Could you check a few things on this model? Use its own coordinates, in mm. A direction names the side the tool comes from. Round coordinates to 2 decimals unless told otherwise and drop trailing zeros. Write each loop counter-clockwise with the first axis right and the second up, starting at its lowest first coordinate (ties: lowest second). Pieces come first, ordered by that corner, then holes.
Autodesk Fusion 360 part; units mm, degrees
sketch "Sketch1" plane through (0, 0, 0) normal (0, 0, 1) x (1, 0, 0)
  circle A0 centre (0, 0) radius 10
  line L0 (-12.5, 12.5) -> (12.5, 12.5)
  line L1 (12.5, 12.5) -> (12.5, -12.5)
  line L2 (12.5, -12.5) -> (-12.5, -12.5)
  line L3 (-12.5, -12.5) -> (-12.5, 12.5)
  line L4 (-12.5, 6.25) -> (12.5, 6.25)
  line L5 (12.5, 6.25) -> (12.5, -6.25)
  line L6 (12.5, -6.25) -> (-12.5, -6.25)
  line L7 (-12.5, -6.25) -> (-12.5, 6.25)
  circle A1 centre (0, 0) radius 5
  dimension "d1" = 20
  dimension "d2" = 25
  dimension "d3" = 25
  dimension "d4" = 12.5
  dimension "d5" = 12.5
  dimension "d6" = 25
  dimension "d7" = 12.5
  dimension "d8" = 6.25
  dimension "d9" = 10
extrude "Extrude1" add sketch "Sketch1" along normal blind 40 contours A0 L4 | A0 L0 L1 L3 L4 | A0 L1 L2 L3 L6 | A0 L6 makes body 1 at (-4.1667, 6.25, 13.3333) makes body 2 at (4.1667, -6.25, 13.3333)
extrude "Extrude2" add sketch "Sketch1" against normal blind 20 contours A0 L4 L6 | A0 L4 | A0 L6 bodies 1 2
extrude "Extrude3" add sketch "Sketch1" along normal blind 10 contours A0 L4 L6 | A0 L1 L4 L5 L6 | A0 L3 L4 L6 L7 bodies 1
sketch "Sketch2" plane through (0, 12.5, 0) normal (0, 1, 0) x (-1, 0, 0)
  line L0 (-12.5, 0) -> (12.5, 0)
  line L1 (12.5, 0) -> (12.5, 40)
  line L2 (12.5, 40) -> (-12.5, 40)
  line L3 (-12.5, 40) -> (-12.5, 0)
  circle A0 centre (0, 27.5) radius 5
  line L4 (12.5, 0) -> (-12.5, 0)
  dimension "d16" = 10
  dimension "d17" = 27.5
extrude "Extrude4" cut sketch "Sketch2" against normal up to surface (25 mm away) contours A0 bodies 1
fillet "Fillet1" radius 12.5 4 edges at (12.5, 9.375, 40) (-12.5, 9.375, 40) (-12.5, -9.375, 40) (12.5, -9.375, 40) on bodies 1
equation "d4 = ( 25 / 2 ) * 1 mm"
equation "d5 = ( 25 / 2 ) * 1 mm"
equation "d8 = ( 12.5 / 2 ) * 1 mm"
Q1. On a 3-axis mill with a long thin cutter (end or side, diameter ignored), from which of +Z, -Z, +X, -X, +Y, -Y can I reach the whole of each face in a straight line? I mean faces 4 (the cylindrical face through (-2.17, -9.76, -9.86)), 5 (the flat face through (0, 6.25, 21)), 6 (the cylindrical face through (-8.94, -9.33, 36.24)). Say none if no direction works.
Q2. Imagine slicing it at D-D, the plane x = -7.5. Write out the boundary of the cut face in (y, z).
Q3. Imagine slicing it at B-B, the plane z = 11.5. Write out the boundary of the cut face in (x, y), then the cut area to 4 significant figures.
Q4. We'd pull the mould along Y, two halves only. Please class faces 1 (the cylindrical face through (8.94, 9.33, 36.24)), 2 (the flat face through (0, -12.5, 20)), 3 (the cylindrical face through (-1.08, 4.88, -5.21)): pulls with the +Y half, pulls with the -Y half, needs draft (parallel to the pull), parting line crosses it, or undercut.
Q5. I'm going to push flat-ended pins straight in: pin 1 Ø12 at (x, z) = (3.5, -4.5) entering from +Y; pin 2 Ø3 at (x, y) = (-3, 2) entering from +Z. Where does each tip first touch, or does it pass through?
Q6. Imagine slicing it at C-C, the plane z = 29. Write out the boundary of the cut face in (x, y).
Q7. If I drill on L1, parallel to Y at x = 2.5, z = 10.5; L2, parallel to Z at x = 0, y = -7.75; L3, parallel to Z at x = 11.5, y = 0.5, over which ranges is the centre line in solid material (lowest first)?
Q8. Imagine slicing it at A-A, the plane y = 0. Write out the boundary of the cut face in (x, z), then the cut area to 3 significant figures.
Results found:
1. face 4: -Z
1. face 5: +Z, +X, -X
1. face 6: +Z, -X, +Y, -Y
2. outline: (-12.5, 0) - (-6.61, 0) - (-6.61, -20) - (6.61, -20) - (6.61, 0) - (12.5, 0) - (12.5, 37.5) - (6.25, 37.5) - (6.25, 10) - (-6.25, 10) - (-6.25, 37.5) - (-12.5, 37.5) - close
3. outline: (-12.5, -12.5) - (12.5, -12.5) - (12.5, -6.25) - (-12.5, -6.25) - close; (-12.5, 6.25) - (12.5, 6.25) - (12.5, 12.5) - (-12.5, 12.5) - close
3. area: 312.5 mm2
4. face 1: needs draft
4. face 2: pulls with the -Y half
4. face 3: undercut
5. pin 1: stops at y = 12.5
5. pin 2: stops at z = 10
6. outline: (-12.41, -12.5) - (-4.77, -12.5) - (-4.77, -6.25) - (-12.41, -6.25) - close; (-12.41, 6.25) - (-4.77, 6.25) - (-4.77, 12.5) - (-12.41, 12.5) - close; (4.77, -12.5) - (12.41, -12.5) - (12.41, -6.25) - (4.77, -6.25) - close; (4.77, 6.25) - (12.41, 6.25) - (12.41, 12.5) - (4.77, 12.5) - close
7. L1: y = -12.5 to -6.25, 6.25 to 12.5
7. L2: z = -20 to 22.5, 32.5 to 40
7. L3: z = 0 to 10
8. outline: (-12.5, 0) - (-10, 0) - (-10, -20) - (-5, -20) - (-5, 10) - (-12.5, 10) - close; (5, -20) - (10, -20) - (10, 0) - (12.5, 0) - (12.5, 10) - (5, 10) - close
8. area: 350 mm2
